Autodesk Inventor part; units mm, degrees
ref_plane "YZ Plane" through (0, 0, 0) normal (1, 0, 0) x (0, 1, 0)
ref_plane "XZ Plane" through (0, 0, 0) normal (0, 1, 0) x (-1, 0, 0)
ref_plane "XY Plane" through (0, 0, 0) normal (0, 0, 1) x (1, 0, 0)
sketch "草圖1" plane through (0, 0, 0) normal (0, 0, 1) x (1, 0, 0)
  circle A0 centre (0, 0) radius 31.05
  dimension "d0" = 62.1
extrude "擠出1" add sketch "草圖1" along normal blind 5
sketch "草圖2" plane through (0, 0, 5) normal (0, 0, 1) x (1, 0, 0)
  circle A0 centre (0, 0) radius 18.85
  dimension "d3" = 37.7
extrude "擠出2" add sketch "草圖2" along normal blind 2
sketch "草圖3" plane through (0, 0, 0) normal (0, 0, -1) x (-1, 0, 0)
  circle A0 centre (0, 0) radius 20
  dimension "d6" = 40
extrude "擠出3" add sketch "草圖3" along normal blind 0.5
sketch "草圖4" plane through (0, 0, 7) normal (0, 0, 1) x (1, 0, 0)
  circle A0 centre (0, 0) radius 15
  dimension "d9" = 30
extrude "擠出4" cut sketch "草圖4" against normal blind 7.5
chamfer "倒角1" distance 4 angle 45 1 edges at (-31.05, 0, 5)
chamfer "倒角2" distance 0.3 angle 45 2 edges at (-15, 0, 7) (-15, 0, -0.5)
properties part number "KMB602PT-機械油封墊片"
The listing builds one solid part. Answer for the finished solid, in the listing's coordinates (mm). A direction names the side the tool comes from. Round coordinates to 2 decimals unless told otherwise and drop trailing zeros. Write each loop counter-clockwise with the first axis right and the second up, starting at its lowest first coordinate (ties: lowest second). Pieces come first, ordered by that corner, then holes. Notation, with made-up numbers: M 73.5,-39 L 126.5,-39 A13 cw 126.5,-30 Z; hole C -9,-31.75 d5. An arc over 180 degrees is marked long. Write each question's results on one line, items separated by ' | '. Start each with the question number.
Item 1: Find section C-C on z = 2. Write down the section's boundary in (x, y), and give its area (3 significant figures).
Item 2: Which of the six approach directions +Z, -Z, +X, -X, +Y, -Y give full straight-line access (tool end or side, diameter ignored) to faces 4 (the cylindrical face through (4.336, 19.524, -0.246)), 5 (the cylindrical face through (-24.64, 18.893, 0.493))?
Item 3: The mould has two halves that part along Y. Classify faces 1 (the flat face through (-18.4, -5.6, 5)), 2 (the cylindrical face through (-14.985, 0.66, 3.298)), 3 (the cylindrical face through (-4.1, 18.4, 6)): +Y half, -Y half, draft (parallel to the pull), parting line (faces both ways), or undercut.
Item 4: Given pin 1 Ø1 at (y, z) = (-17, 4) entering from -X; pin 2 Ø16 at (x, y) = (2, 3.5) entering from +Z; pin 3 Ø4 at (y, z) = (-2.5, 4.5) entering from +X; pin 4 Ø2 at (x, z) = (21.5, 1.5) entering from +Y, each flat-ended and moving along its own axis, determine where each tip first touches the part or whether it passes through.
Item 5: Straight lines are drawn through the part: probe 1 along Z at (x, y) = (20, -2.5); probe 2 along Y at (x, z) = (10.5, 6.25); probe 3 along X at (y, z) = (3, 1.5). For each, find the intervals that lie inside material, in ascending order.
Item 6: Find section A-A on x = 0. Write down the section's boundary in (y, z), and give its area (3 significant figures).
Answer block:
1) outline: C 0,0 d60.1; hole C 0,0 d30 | area: 2,130 mm²
2) face 4: -Z | face 5: +Z, -Z
3) face 1: draft | face 2: undercut | face 3: parting line
4) pin 1: stops at x = -23.04 | pin 2: passes through | pin 3: stops at x = 29.45 | pin 4: stops at y = 23.2
5) probe 1: z = 0 to 5 | probe 2: y = -15.65 to -10.71, 10.71 to 15.65 | probe 3: x = -30.4 to -14.7, 14.7 to 30.4
6) outline: M -31.05,0 L -20,0 L -20,-0.5 L -15.3,-0.5 L -15,-0.2 L -15,6.7 L -15.3,7 L -18.85,7 L -18.85,5 L -27.05,5 L -31.05,1 Z; M 15,-0.2 L 15.3,-0.5 L 20,-0.5 L 20,0 L 31.05,0 L 31.05,1 L 27.05,5 L 18.85,5 L 18.85,7 L 15.3,7 L 15,6.7 Z | area: 165 mm²
